```python
from build123d import *

# Parameters (mm, degrees)
F0_W     = 119.084648788
F0_H     = 67.9154656827
F1_DEPTH = 25.4
F3_DEPTH = 25.4
F4_W     = 119.084648788
F4_H     = 16.1182302982
F5_DEPTH = 27.94
F7_DEPTH = 25.4
F9_DEPTH = 25.4
F12_D    = 21.59


with BuildPart() as f1:
    # F0 (on Top) → F1 (new body)
    with BuildSketch(Plane.XY):
        with Locations((0.348880887, -8.3731394261)):
            Rectangle(F0_W, F0_H)
    extrude(amount=F1_DEPTH)

    # F2 (on face) → F3 (cut)
    with BuildSketch(Plane.XZ.offset(42.3308722675)):
        Polygon((-43.3775149286, 13.3852101862), (-27.7941711247, 0), (21.2817266583, 0), (33.3762653172, 13.3852101862), align=None)
    extrude(amount=-F3_DEPTH, mode=Mode.SUBTRACT)

    # F4 (on face) → F5 (join)
    with BuildSketch(Plane.XY.offset(25.4)):
        with Locations((0.348880887, 17.5254782662)):
            Rectangle(F4_W, F4_H)
    extrude(amount=F5_DEPTH)

    # F6 (on face) → F7 (cut)
    with BuildSketch(Plane.XZ.offset(-9.4663631171)):
        Polygon((-59.193443507, 39.37), (-48.261847347, 53.34), (-59.193443507, 53.34), align=None)
    extrude(amount=-F7_DEPTH, mode=Mode.SUBTRACT)

    # F8 (on face) → F9 (cut)
    with BuildSketch(Plane.XZ.offset(-9.4663631171)):
        Polygon((59.891205281, 53.34), (48.4944358468, 53.34), (59.891205281, 37.4465435743), align=None)
    extrude(amount=-F9_DEPTH, mode=Mode.SUBTRACT)

    # F12 (through all)
    with Locations(Plane.XY.offset(25.4)):
        with Locations((0, -15.5321601778)):
            Hole(F12_D / 2)


solid = f1.part
```
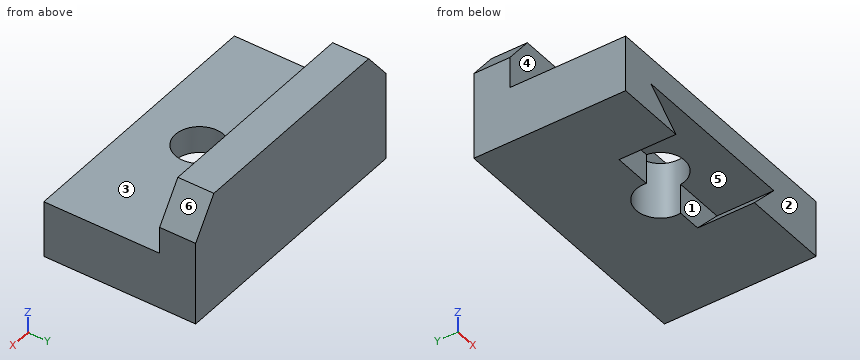
Geometry check sheet. Reference: the model listing, model coordinates, mm. Face numbers are marked on the shaded views. A direction names the side the tool comes from. Round coordinates to 2 decimals unless told otherwise and drop trailing zeros. Loops run counter-clockwise (first coordinate to the right, second up) from the corner with the lowest first, then second, coordinate; pieces in that order, holes last. Notation, with made-up numbers: (47, -34.5) - (54, -34.5) arc R34 cw to (54, 3.5) - close; hole circle Ø10 at (75, 46.25). An arc over 180 degrees is marked (long way). Write each question's results on one line, items separated by ' | '. Start each with the question number.
Q1. Access from +Z, -Z, +X, -X, +Y, -Y to the whole of each face (thin tool, end or side, straight path). Record for the marked faces 4, 5 and 6.
Q2. Cross-section at A-A on x = 0. Enter the section's corners in (y, z), and give its area (3 significant figures).
Q3. Release check for a two-part mould opening along Z. For the marked faces 1, 2 and 3 record: +Z half, -Z half, draft (parallel to the pull), parting line (faces both ways), or undercut.
Q4. Cross-section at C-C on x = -19. Enter the section's corners in (y, z).
Q5. Gauge pin test, flat ends, axial feed: P1, Ø4, axis at x = 20.5, z = 9.5, coming from the -Y side; P2, Ø14, axis at x = -7.5, z = 34.5, coming from the -Y side; P3, Ø3, axis at x = -44.5, y = -17.5, coming from the +Z side. Record the tip position at first contact, or that the pin passes through.
Q6. Thickness scan on line 1 (Y direction, x = 0, z = 16.5); line 2 (Z direction, x = 11, y = -30); line 3 (Z direction, x = 7, y = 7). Record the ranges inside material, lowest first. Write a range as [from, to].
Q7. Cross-section at D-D on y = -31. Enter the section's corners in (x, z), and give its area (3 significant figures).
Q8. Cross-section at B-B on y = -10.5. Enter the section's corners in (x, z), and give its area (3 significant figures).
Answers below:
1) face 4: +Z, +X, -X, -Y | face 5: -Y | face 6: +Z, +X, +Y, -Y
2) outline: (-42.33, 13.39) - (-26.33, 13.39) - (-26.33, 25.4) - (-42.33, 25.4) - close; (-4.74, 0) - (25.58, 0) - (25.58, 53.34) - (9.47, 53.34) - (9.47, 25.4) - (-4.74, 25.4) - close | area: 1,410 mm²
3) face 1: undercut | face 2: draft | face 3: +Z half
4) outline: (-42.33, 13.39) - (-16.93, 13.39) - (-16.93, 0) - (25.58, 0) - (25.58, 53.34) - (9.47, 53.34) - (9.47, 25.4) - (-42.33, 25.4) - close
5) P1: stops at y = -16.93 | P2: stops at y = 9.47 | P3: stops at z = 25.4
6) line 1: y = [-42.33, -26.33], [-4.74, 25.58] | line 2: z = [13.39, 25.4] | line 3: z = [0, 25.4]
7) outline: (-59.19, 0) - (-27.79, 0) - (-43.38, 13.39) - (33.38, 13.39) - (21.28, 0) - (59.89, 0) - (59.89, 25.4) - (-59.19, 25.4) - close | area: 2,180 mm²
8) outline: (-59.19, 0) - (-9.55, 0) - (-9.55, 25.4) - (-59.19, 25.4) - close; (9.55, 0) - (59.89, 0) - (59.89, 25.4) - (9.55, 25.4) - close | area: 2,540 mm²
